Here's how the part is built. I have some questions about the finished solid (model axes, mm). Face numbers are marked on the shaded views. A direction names the side the tool comes from. Coordinates: 2 decimals unless noted, no trailing zeros. Loops run counter-clockwise (first coordinate to the right, second up) from the corner with the lowest first, then second, coordinate; pieces in that order, holes last. Notation, with made-up numbers: (-5.75, 24) - (38.25, 24) arc R16 cw to (38.25, 44) - close; hole circle Ø2 at (58, 12). An arc over 180 degrees is marked (long way). Use a Markdown table: item, result.
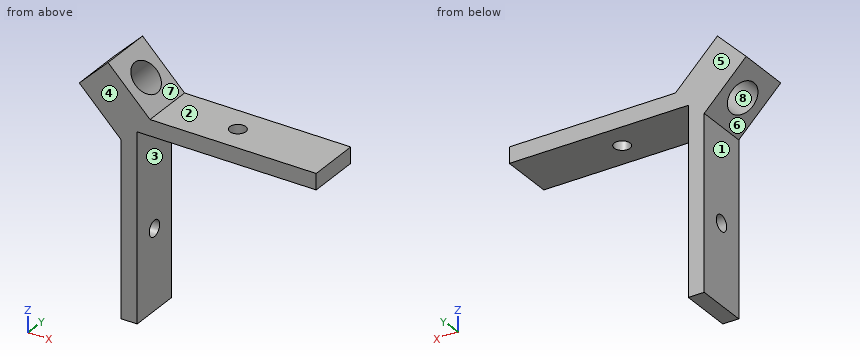
```python
from build123d import *

# Parameters (mm, degrees)
BOSS_EXTRUDE1_DEPTH = 10
SKETCH3_R           = 1.5
CUT_EXTRUDE1_DEPTH  = 30
SKETCH4_R           = 1.5
CUT_EXTRUDE2_DEPTH  = 30
CUT_EXTRUDE5_DEPTH  = 30
SKETCH9_R           = 3
CUT_EXTRUDE6_DEPTH  = 30


with BuildPart() as part:
    # Sketch1 → Boss-Extrude1 (new body)
    with BuildSketch(Plane(origin=(0, 0, 0), x_dir=(1, 0, 0), z_dir=(0, 1, 0))):
        Polygon((1.311744675, 2.415195475), (1.311744675, 35), (4.311744675, 35), (4.311744675, 0), (38, 0), (38, -3), (6.726940148, -3), (6.726940148, -11.726940148), (3.191406243, -15.262474054), (-10.950729381, -1.120338431), (-7.415195475, 2.415195475), align=None)
    extrude(amount=BOSS_EXTRUDE1_DEPTH)

    # Sketch3 → Cut-Extrude1 (cut)
    with BuildSketch(Plane.XY.offset(3)):
        with Locations((20, 5)):
            Circle(SKETCH3_R)
    extrude(amount=-CUT_EXTRUDE1_DEPTH, mode=Mode.SUBTRACT)

    # Sketch4 → Cut-Extrude2 (cut)
    with BuildSketch(Plane.ZY.offset(-1.311744675)):
        with Locations((-20, 5)):
            Circle(SKETCH4_R)
    extrude(amount=-CUT_EXTRUDE2_DEPTH, mode=Mode.SUBTRACT)

    # Sketch8 → Cut-Extrude5 (cut)
    with BuildSketch(Plane(origin=(0, 10, 0), x_dir=(1, 0, 0), z_dir=(0, 1, 0))):
        Polygon((1.311744675, 2.415195475), (-7.06515363, -5.961702829), (-14.174938383, 1.148081923), (-5.798040078, 9.524980228), align=None)
        Polygon((6.726940148, -3), (-1.172063832, -10.89900398), (4.537107227, -16.608175039), (12.436111207, -8.709171058), align=None)
    extrude(amount=-CUT_EXTRUDE5_DEPTH, mode=Mode.SUBTRACT)

    # Sketch9 → Cut-Extrude6 (cut)
    with BuildSketch(Plane(origin=(-0.5517254, 0, -0.5517254), x_dir=(-0.7071067811865474, 0, 0.7071067811865477), z_dir=(-0.7071067811865477, 0, -0.7071067811865474))):
        with Locations((3, 5)):
            Circle(SKETCH9_R)
    extrude(amount=-CUT_EXTRUDE6_DEPTH, mode=Mode.SUBTRACT)


solid = part.part
```
Q1. I want a section at B-B, the plane x = 20. Write out the boundary of the cut face in (y, z), then the cut area to 3 significant figures.
Check values:
| item | result |
|---|---|
| outline | (0, 0) - (3.5, 0) - (3.5, 3) - (0, 3) - close; (6.5, 0) - (10, 0) - (10, 3) - (6.5, 3) - close |
| area | 21.0 mm^2 |
Q2. I want a section at A-A, the plane z = -20. Write out the boundary of the cut face in (x, y).
Check values:
| item | result |
|---|---|
| outline | (1.31, 0) - (4.31, 0) - (4.31, 3.5) - (1.31, 3.5) - close; (1.31, 6.5) - (4.31, 6.5) - (4.31, 10) - (1.31, 10) - close |
Q3. I want a section at C-C, the plane y = 5. Write out the boundary of the cut face in (x, z).
Check values:
| item | result |
|---|---|
| outline | (-6.59, 5.48) - (-4.79, 3.69) - (0.62, 9.11) - (-1.17, 10.9) - close; (-0.55, -0.55) - (1.31, -2.42) - (1.31, -18.5) - (4.31, -18.5) - (4.31, 0) - (18.5, 0) - (18.5, 3) - (6.73, 3) - (4.86, 4.86) - close; (1.31, -35) - (4.31, -35) - (4.31, -21.5) - (1.31, -21.5) - close; (21.5, 0) - (38, 0) - (38, 3) - (21.5, 3) - close |
Q4. If we mould it in two halves opening along Z, with no side actions, what happens to the marked faces 5, 6, 7 and 8? For each: pulls with the +Z half, pulls with the -Z half, needs draft (parallel to the pull), parting line crosses it, or undercut.
Check values:
| item | result |
|---|---|
| face 5 | needs draft |
| face 6 | pulls with the -Z half |
| face 7 | pulls with the +Z half |
| face 8 | undercut |
Q5. Please list where these lines run through material, in increasing order: L1, parallel to Y at x = 3.15, z = -20; L2, parallel to X at y = 5.75, z = -12; L3, parallel to Z at x = 26.5, y = 2.5. Write a range as from..to.
Check values:
| item | result |
|---|---|
| L1 | 0..3.5, 6.5..10 |
| L2 | 1.31..4.31 |
| L3 | 0..3 |
Q6. I want a section at D-D, the plane z = -15. Write out the boundary of the cut face in (x, y).
Check values:
| item | result |
|---|---|
| outline | (1.31, 0) - (4.31, 0) - (4.31, 10) - (1.31, 10) - close |
Q7. Will these pins go through, and if not, where does the flat tip stop? P1, Ø1, axis at x = 13, y = 2, coming from the -Z side; P2, Ø3.5, axis at x = 20, y = 5, coming from the +Z side; P3, Ø6, axis at y = 1.5, z = -13, coming from the +X side.
Check values:
| item | result |
|---|---|
| P1 | z = 0 |
| P2 | z = 3 |
| P3 | x = 4.31 |
Q8. Which directions (+Z, -Z, +X, -X, +Y, -Y) give clear straight access to the entire face, cutting with the end or side of a thin tool? Please do the marked faces 1, 2, 3 and 4.
Check values:
| item | result |
|---|---|
| face 1 | -Z, -X, +Y, -Y |
| face 2 | +Z, +X, +Y, -Y |
| face 3 | -Z, +X, +Y, -Y |
| face 4 | +Z, -Z, +X, -X, -Y |
